Here's how the part is built. I have some questions about the finished solid (model axes, mm). A direction names the side the tool comes from. Round coordinates to 2 decimals unless told otherwise and drop trailing zeros. Order: outer loops, then holes, each group sorted by start corner. A loop starts at its lowest first (then second) coordinate and runs counter-clockwise, first axis right, second up.
```python
from build123d import *

# Parameters (mm, degrees)
BOSS_EXTRUDE1_DEPTH      = 410
BOSS_EXTRUDE1_DEPTH_BACK = 20
F_3_0_3_DIAMETER_HOLE1_D = 3


with BuildPart() as part:
    # Sketch1 → Boss-Extrude1 (new, two sides: drawn at the far end of the back side and taken through both)
    with BuildSketch(Plane.XY.offset(-BOSS_EXTRUDE1_DEPTH_BACK)):
        Polygon((0, 5.602318429), (0, 35.602318429), (2, 35.602318429), (2, 7.602318429), (30, 7.602318429), (30, 5.602318429), align=None)
    extrude(amount=BOSS_EXTRUDE1_DEPTH + BOSS_EXTRUDE1_DEPTH_BACK)

    # Ø3.0 (3) Diameter Hole1 (through all)
    with Locations(Plane(origin=(0, 136.46431451, 221.32004832), x_dir=(0, 1, 0), z_dir=(-1, 0, 0))):
        with Locations((-122.861996081, -170.67995168), (-108.861996081, -170.67995168), (215.138003919, -170.67995168), (201.138003919, -170.67995168)):
            Hole(F_3_0_3_DIAMETER_HOLE1_D / 2)


solid = part.part
```
1. If we section it at C-C, the plane x = 16.5: Write out the boundary of the cut face in (y, z), and give its area (3 significant figures).
Evaluation:
outline: (5.6, -20) - (7.6, -20) - (7.6, 410) - (5.6, 410) - close
area: 860 mm2
2. If we section it at B-B, the plane y = 21.25: Write out the boundary of the cut face in (x, z).
Evaluation:
outline: (0, -20) - (2, -20) - (2, 410) - (0, 410) - close
3. I'm going to push flat-ended pins straight in: P1, Ø1.5, axis at y = 9.5, z = 205.5, coming from the +X side; P2, Ø1, axis at x = 8, z = 206.5, coming from the +Y side. Where does each tip first touch, or does it pass through?
Evaluation:
P1: stops at x = 2
P2: stops at y = 7.6
4. I need wall thicknesses on probe 1 along Y at (x, z) = (0.5, 392); probe 2 along X at (y, z) = (22, 51); probe 3 along Y at (x, z) = (17.5, 203). Which ranges of each line are inside material? Lowest first, please.
Evaluation:
probe 1: y = 5.6 to 12.1, 15.1 to 26.1, 29.1 to 35.6
probe 2: x = 0 to 2
probe 3: y = 5.6 to 7.6
5. If we section it at A-A, the plane z = 369: Write out the boundary of the cut face in (x, y), and give its area (3 significant figures).
Evaluation:
outline: (0, 5.6) - (30, 5.6) - (30, 7.6) - (2, 7.6) - (2, 35.6) - (0, 35.6) - close
area: 116 mm2
6. On a 3-axis mill with a long thin cutter (end or side, diameter ignored), from which of +Z, -Z, +X, -X, +Y, -Y can I reach the whole of each face in a straight line? I mean faces 1 (the flat face through (0, 20, 192)), 2 (the flat face through (2, 22, 192)). Say none if no direction works.
Evaluation:
face 1: +Z, -Z, -X, +Y, -Y
face 2: +Z, -Z, +X, +Y
